Here's how the part is built. I have some questions about the finished solid (model axes, mm). Face numbers are marked on the shaded views. Round coordinates to 2 decimals unless told otherwise and drop trailing zeros. Write each loop counter-clockwise with the first axis right and the second up, starting at its lowest first coordinate (ties: lowest second). Pieces come first, ordered by that corner, then holes. Notation, with made-up numbers: M -27.75,67 L 27.25,67 A18 cw 27.25,74 Z; hole C 72,9 d11. An arc over 180 degrees is marked long. Use one line per item in the form item = value. Start each with the question number.
Q1. I want a section at D-D on x = 25. List the corners of the cut face in (y, z) for me, and give its area (3 significant figures).
Q2. I'm going to push flat-ended pins straight in: pin 1 Ø7.5 at (x, z) = (17.5, 17) entering from -Y; pin 2 Ø1 at (y, z) = (-8, 37) entering from +X; pin 3 Ø7.5 at (x, z) = (16, 14.5) entering from +Y (3 decimals). Where does each tip first touch, or does it pass through?
Q3. I want a section at A-A on y = 0. List the corners of the cut face in (x, z) for me, and give its area (3 significant figures).
Q4. I want a section at B-B on x = -18. List the corners of the cut face in (y, z) for me, and give its area (4 significant figures).
Q5. I want a section at C-C on z = 20.5. State how many separate pieces and enclosed holes the cut face has, and give its area (3 significant figures).
Q6. I need wall thicknesses on line 1 along Y through (x, z) = (0, 33.5); line 2 along X through (y, z) = (-3.5, 3); line 3 along X through (y, z) = (-20, 25.5). Which ranges of each line are inside material? Lowest first, please. Write a range as from..to.
Q7. We'd pull the mould along X, two halves only. Please class the marked faces 1, 2, 3 and 4: +X half, -X half, draft (parallel to the pull), parting line (faces both ways), or undercut.
```python
from build123d import *

# Parameters (mm, degrees)
F0_R            = 30
F0_R_2          = 15
F1_DEPTH        = 50
F2_W            = 12.7
F2_H            = 12.7
F3_DEPTH        = 50.001
F3_COPIES_COUNT = 4
F4_W            = 9.525
F4_H            = 9.525
F5_DEPTH        = 50.001
F5_COPIES_COUNT = 4


# Not quite as in the source:
# - a pattern or mirror of a feature is missing from the dataset's text; its kind, count and spacing are read off the source's solid


with BuildPart() as f1:
    # F0 (on Top) → F1 (new body)
    with BuildSketch(Plane.XY):
        Circle(F0_R)
        Circle(F0_R_2, mode=Mode.SUBTRACT)
    extrude(amount=F1_DEPTH)

    # F2 (on face) → F3 (cut, through all)
    with BuildSketch(Plane.XY.offset(50)):
        with Locations((0, 22.5)):
            Rectangle(F2_W, F2_H)
    f3 = extrude(amount=-F3_DEPTH, mode=Mode.SUBTRACT)

    # F3_copies: F3 ×4 about axis
    f3_copies_axis = Axis((0, 0, 0), (0, 0, 1))
    for i in range(1, F3_COPIES_COUNT):
        add(f3.rotate(f3_copies_axis, i * 360 / F3_COPIES_COUNT), mode=Mode.SUBTRACT)

    # F4 (on face) → F5 (cut, through all)
    with BuildSketch(Plane.XY.offset(50)):
        with Locations((-15.9099025767, 15.9099025767)):
            Rectangle(F4_W, F4_H)
    f5 = extrude(amount=-F5_DEPTH, mode=Mode.SUBTRACT)

    # F5_copies: F5 ×4 about axis
    f5_copies_axis = Axis((0, 0, 0), (0, 0, 1))
    for i in range(1, F5_COPIES_COUNT):
        add(f5.rotate(f5_copies_axis, i * 360 / F5_COPIES_COUNT), mode=Mode.SUBTRACT)


solid = f1.part
```
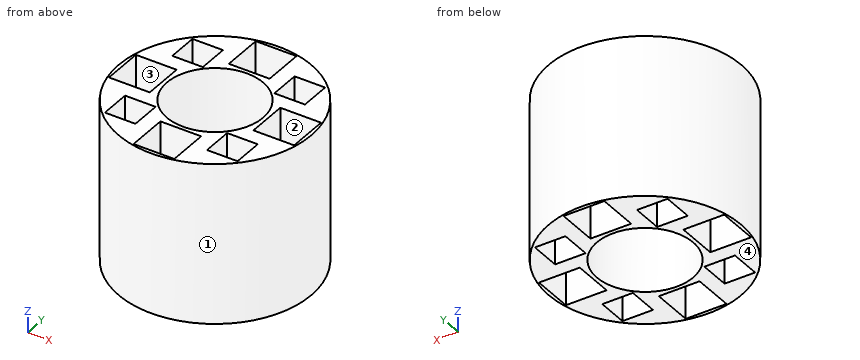
Reported:
q1.outline = M -16.58,0 L -6.35,0 L -6.35,50 L -16.58,50 Z; M 6.35,0 L 16.58,0 L 16.58,50 L 6.35,50 Z
q1.area = 1,020 mm^2
q2.pin_1 = -26.66
q2.pin_2 = 29.05
q2.pin_3 = 27.385
q3.outline = M -30,0 L -28.85,0 L -28.85,50 L -30,50 Z; M -16.15,0 L -15,0 L -15,50 L -16.15,50 Z; M 15,0 L 16.15,0 L 16.15,50 L 15,50 Z; M 28.85,0 L 30,0 L 30,50 L 28.85,50 Z
q3.area = 230 mm^2
q4.outline = M -24,0 L -20.67,0 L -20.67,50 L -24,50 Z; M -11.15,0 L -6.35,0 L -6.35,50 L -11.15,50 Z; M 6.35,0 L 11.15,0 L 11.15,50 L 6.35,50 Z; M 20.67,0 L 24,0 L 24,50 L 20.67,50 Z
q4.area = 812.5 mm^2
q5.separate_pieces = 1
q5.enclosed_holes = 9
q5.area = 1,110 mm^2
q6.line_1 = -30..-28.85, -16.15..-15, 15..16.15, 28.85..30
q6.line_2 = -29.8..-28.85, -16.15..-14.59, 14.59..16.15, 28.85..29.8
q6.line_3 = -22.36..-20.67, -11.15..-6.35, 6.35..11.15, 20.67..22.36
q7.face_1 = parting line
q7.face_2 = undercut
q7.face_3 = undercut
q7.face_4 = draft
